Can you work these out from the model? Positions are in its coordinate system, mm. Face numbers are marked on the shaded views. A direction names the side the tool comes from. Give positions to 0.01 mm unless a question says otherwise; leave off trailing zeros. Order: outer loops, then holes, each group sorted by start corner. A loop starts at its lowest first (then second) coordinate and runs counter-clockwise, first axis right, second up. Notation, with made-up numbers: (-37.75, 55.5) - (-27.75, 55.5) arc R33 ccw to (-27.75, 91.5) - close; hole circle Ø11 at (-6, 45). An arc over 180 degrees is marked (long way). Answer as a JSON object with one key per item and string values.
```python
from build123d import *
from OCP.BRepFilletAPI import BRepFilletAPI_MakeChamfer

# Parameters (mm, degrees)
SKETCH1_W           = 30
SKETCH1_H           = 26.5
BOSS_EXTRUDE1_DEPTH = 12
FILLET1_R           = 3
FILLET2_R           = 1
SKETCH2_R           = 3.75
CUT_EXTRUDE1_DEPTH  = 5
SKETCH3_R           = 3
BOSS_EXTRUDE2_DEPTH = 5
SKETCH4_R           = 1.75
CUT_EXTRUDE2_DEPTH  = 0.75
CHAMFER1_SIZE       = 0.75
SKETCH5_W           = 2.9
SKETCH5_H           = 10
BOSS_EXTRUDE3_DEPTH = 10
CHAMFER2_SIZE       = 4
CHAMFER2_SIZE2      = 2
BOSS_EXTRUDE4_DEPTH = 6.2
SKETCH7_W           = 30
SKETCH7_H           = 24
BOSS_EXTRUDE5_DEPTH = 2
FILLET3_R           = 3
SKETCH8_W           = 11.5
SKETCH8_H           = 7.5
CUT_EXTRUDE3_DEPTH  = 5


with BuildPart() as part:
    # Sketch1 → Boss-Extrude1 (new body)
    with BuildSketch(Plane.XY):
        Rectangle(SKETCH1_W, SKETCH1_H)
    extrude(amount=BOSS_EXTRUDE1_DEPTH)

    # Fillet1
    fillet1_edges = [part.edges().sort_by_distance(p)[0] for p in [
        (-15, -13.25, 6),
        (15, -13.25, 6),
        (15, 13.25, 6),
        (-15, 13.25, 6),
    ]]
    fillet(fillet1_edges, radius=FILLET1_R)

    # Fillet2
    fillet2_edges = [part.edges().sort_by_distance(p)[0] for p in [
        (15, 0, 12),
        (0, -13.25, 12),
        (-15, 0, 12),
        (0, 13.25, 12),
        (-14.121320344, 12.371320344, 12),
        (14.121320344, 12.371320344, 12),
        (-14.121320344, -12.371320344, 12),
        (14.121320344, -12.371320344, 12),
    ]]
    fillet(fillet2_edges, radius=FILLET2_R)

    # Sketch2 → Cut-Extrude1 (cut)
    with BuildSketch(Plane.XY.offset(12)):
        with Locations((0, -2.75)):
            Circle(SKETCH2_R)
    extrude(amount=-CUT_EXTRUDE1_DEPTH, mode=Mode.SUBTRACT)

    # Sketch3 → Boss-Extrude2 (add)
    with BuildSketch(Plane.XY.offset(7)):
        with Locations((0, -2.75)):
            Circle(SKETCH3_R)
    extrude(amount=BOSS_EXTRUDE2_DEPTH)

    # Sketch4 → Cut-Extrude2 (cut)
    with BuildSketch(Plane.XY.offset(12)):
        with Locations((0, -2.75)):
            Circle(SKETCH4_R)
    extrude(amount=-CUT_EXTRUDE2_DEPTH, mode=Mode.SUBTRACT)

    # Chamfer1
    chamfer1_edges = [part.edges().sort_by_distance(p)[0] for p in [
        (-1.75, -2.75, 12),
    ]]
    chamfer(chamfer1_edges, length=CHAMFER1_SIZE - 0.0001)  # a hair under: the kernel refuses the full size

    # Sketch5 → Boss-Extrude3 (add)
    with BuildSketch(Plane(origin=(0, 0, 0), x_dir=(-1, 0, 0), z_dir=(0, 0, -1))):
        with Locations((-4.55, 6.25)):
            Rectangle(SKETCH5_W, SKETCH5_H)
        with Locations((4.55, 6.25)):
            Rectangle(SKETCH5_W, SKETCH5_H)
    extrude(amount=BOSS_EXTRUDE3_DEPTH)

    # Chamfer2: one chamfer whose edges measure the first distance from different faces: ONE call of the kernel's chamfer builder (chamfer() names one face for all edges)
    chamfer2_edges_1 = [part.edges().sort_by_distance(p)[0] for p in [
        (-4.55, 1.25, -10),
    ]]
    chamfer2_side_1 = [part.faces().sort_by_distance(p)[0] for p in [
        (-4.55, 1.25, -5),
    ]]
    chamfer2_edges_2 = [part.edges().sort_by_distance(p)[0] for p in [
        (4.55, 1.25, -10),
    ]]
    chamfer2_side_2 = [part.faces().sort_by_distance(p)[0] for p in [
        (4.55, 1.25, -5),
    ]]
    chamfer2_edges_3 = [part.edges().sort_by_distance(p)[0] for p in [
        (4.55, 11.25, -10),
    ]]
    chamfer2_side_3 = [part.faces().sort_by_distance(p)[0] for p in [
        (4.55, 11.25, -5),
    ]]
    chamfer2_edges_4 = [part.edges().sort_by_distance(p)[0] for p in [
        (-4.55, 11.25, -10),
    ]]
    chamfer2_side_4 = [part.faces().sort_by_distance(p)[0] for p in [
        (-4.55, 11.25, -5),
    ]]
    chamfer2 = BRepFilletAPI_MakeChamfer(part.part.solid().wrapped)
    for e in chamfer2_edges_1:
        chamfer2.Add(CHAMFER2_SIZE, CHAMFER2_SIZE2, e.wrapped, chamfer2_side_1[0].wrapped)  # the first distance lies on this face
    for e in chamfer2_edges_2:
        chamfer2.Add(CHAMFER2_SIZE, CHAMFER2_SIZE2, e.wrapped, chamfer2_side_2[0].wrapped)  # the first distance lies on this face
    for e in chamfer2_edges_3:
        chamfer2.Add(CHAMFER2_SIZE, CHAMFER2_SIZE2, e.wrapped, chamfer2_side_3[0].wrapped)  # the first distance lies on this face
    for e in chamfer2_edges_4:
        chamfer2.Add(CHAMFER2_SIZE, CHAMFER2_SIZE2, e.wrapped, chamfer2_side_4[0].wrapped)  # the first distance lies on this face
    add(Compound.cast(chamfer2.Shape()), mode=Mode.REPLACE)

    # Sketch6 → Boss-Extrude4 (add)
    with BuildSketch(Plane(origin=(-3.1, 0, 0), x_dir=(0, 0, -1), z_dir=(1, 0, 0))):
        Polygon((2, 9.25), (2, 3.25), (6, 1.25), (12, 1.25), (12, 11.25), (6, 11.25), align=None)
    extrude(amount=BOSS_EXTRUDE4_DEPTH)

    # Sketch7 → Boss-Extrude5 (add)
    with BuildSketch(Plane(origin=(0, 0, -12), x_dir=(-1, 0, 0), z_dir=(0, 0, -1))):
        with Locations((0, 1.25)):
            Rectangle(SKETCH7_W, SKETCH7_H)
    extrude(amount=BOSS_EXTRUDE5_DEPTH)

    # Fillet3
    fillet3_edges = [part.edges().sort_by_distance(p)[0] for p in [
        (-15, -10.75, -13),
        (-15, 13.25, -13),
        (15, 13.25, -13),
        (15, -10.75, -13),
    ]]
    fillet(fillet3_edges, radius=FILLET3_R)

    # Sketch8 → Cut-Extrude3 (cut)
    with BuildSketch(Plane(origin=(0, 0, 0), x_dir=(-1, 0, 0), z_dir=(0, 0, -1))):
        with Locations((5.75, -9.5)):
            Rectangle(SKETCH8_W, SKETCH8_H)
        with Locations((-5.75, -9.5)):
            Rectangle(SKETCH8_W, SKETCH8_H)
    extrude(amount=-CUT_EXTRUDE3_DEPTH, mode=Mode.SUBTRACT)


solid = part.part
```
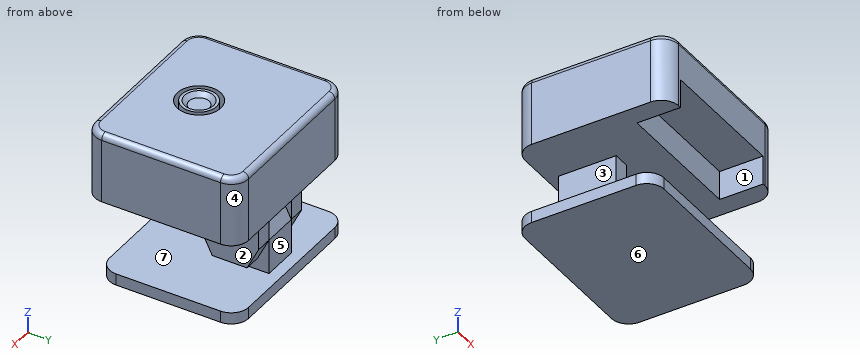
Q1. If we section it at B-B, the plane x = 7.5: Please give me the cut outline in (y, z), then the cut area to 3 significant figures.
Recorded:
{"outline": "(-13.25, 5) - (-5.75, 5) - (-5.75, 0) - (13.25, 0) - (13.25, 11) arc R1 ccw to (12.25, 12) - (-12.25, 12) arc R1 ccw to (-13.25, 11) - close; (-10.75, -14) - (13.25, -14) - (13.25, -12) - (-10.75, -12) - close", "area": "328 mm^2"}
Q2. Which directions (+Z, -Z, +X, -X, +Y, -Y) give clear straight access to the entire face, cutting with the end or side of a thin tool? Please do the marked faces 1, 2 and 3.
Recorded:
{"face 1": "-Y", "face 2": "+X, +Y, -Y", "face 3": "-X, +Y, -Y"}
Q3. I need wall thicknesses on L1, parallel to Y at x = 0, z = 9.6; L2, parallel to X at y = 4, z = -1.75; L3, parallel to Z at x = -1.75, y = 3. Which ranges of each line are inside material? Lowest first, please.
Recorded:
{"L1": "y = -13.25 to -6.5, -5.75 to 0.25, 1 to 13.25", "L2": "x = -6 to -3.1, 3.1 to 6", "L3": "z = -14 to -2.5, 0 to 12"}
Q4. If we section it at A-A, the plane z = 9.75: Please give me the cut outline in (x, y).
Recorded:
{"outline": "(-15, -10.25) arc R3 ccw to (-12, -13.25) - (12, -13.25) arc R3 ccw to (15, -10.25) - (15, 10.25) arc R3 ccw to (12, 13.25) - (-12, 13.25) arc R3 ccw to (-15, 10.25) - close; circle Ø6 at (0, -2.75); hole circle Ø7.5 at (0, -2.75)"}
Q5. I'm going to push flat-ended pins straight in: pin 1 Ø5 at (y, z) = (4, -4) entering from +X; pin 2 Ø5 at (x, z) = (4, -1) entering from +Y; pin 3 Ø2.5 at (x, z) = (4, 2) entering from -Y; pin 4 Ø0.9 at (x, z) = (5, -4) entering from -Y. Where does each tip first touch, or does it pass through?
Recorded:
{"pin 1": "stops at x = 6", "pin 2": "stops at y = 13.25", "pin 3": "stops at y = -5.75", "pin 4": "stops at y = 1.25"}
Q6. We'd pull the mould along Z, two halves only. Please class the marked faces 4, 5, 6 and 7: released by +Z, released by -Z, zero draft, split by the parting line, or undercut.
Recorded:
{"face 4": "zero draft", "face 5": "undercut", "face 6": "released by -Z", "face 7": "undercut"}
Q7. If we section it at D-D, the plane z = 0.5: Please give me the cut outline in (x, y), then the cut area to 3 significant figures.
Recorded:
{"outline": "(-15, -10.25) arc R3 ccw to (-12, -13.25) - (-11.5, -13.25) - (-11.5, -5.75) - (11.5, -5.75) - (11.5, -13.25) - (12, -13.25) arc R3 ccw to (15, -10.25) - (15, 10.25) arc R3 ccw to (12, 13.25) - (-12, 13.25) arc R3 ccw to (-15, 10.25) - close", "area": "615 mm^2"}
